Read the model definition and answer for the solid it produces. Units are mm, in the model's axes. A direction names the side the tool comes from. Give positions to 0.01 mm unless a question says otherwise; leave off trailing zeros. Loops run counter-clockwise (first coordinate to the right, second up) from the corner with the lowest first, then second, coordinate; pieces in that order, holes last. Notation, with made-up numbers: (-36.5, 75) - (21.5, 75) arc R25 ccw to (21.5, 94) - close; hole circle Ø9 at (76.5, -20.5). An arc over 180 degrees is marked (long way). Write item = value, one per line.
```python
from build123d import *

# Parameters (mm, degrees)
SKETCH1_W                      = 52.7
SKETCH1_H                      = 40.2
SKETCH1_W_2                    = 40
SKETCH1_H_2                    = 27.5
BOSS_EXTRUDE1_DEPTH            = 46
SKETCH2_R                      = 1.7
SKETCH2_R_2                    = 3.25
CUT_EXTRUDE1_DEPTH             = 6.35
BOSS_EXTRUDE2_DEPTH            = 242.29
SKETCH4_W                      = 288.29
SKETCH4_H                      = 6.35
BOSS_EXTRUDE3_DEPTH            = 7
SKETCH6_W                      = 288.29
SKETCH6_H                      = 6.35
BOSS_EXTRUDE4_DEPTH            = 7
SKETCH7_W                      = 6.35
SKETCH7_H                      = 25
BOSS_EXTRUDE5_DEPTH            = 7
CUT_EXTRUDE2_REACH             = 297.989
SKETCH9_R                      = 2.5
CUT_EXTRUDE2_DIRECTION_2_REACH = 297.989
CUT_EXTRUDE3_REACH             = 253.822
SKETCH10_R                     = 1.2
SKETCH11_W                     = 21.35
SKETCH11_H                     = 6.8
SKETCH11_W_2                   = 214.59
CUT_EXTRUDE4_DEPTH             = 52.7
SKETCH12_W                     = 6.35
SKETCH12_H                     = 6.35
CUT_EXTRUDE5_DEPTH             = 6.8


with BuildPart() as part:
    # Sketch1 → Boss-Extrude1 (new body)
    with BuildSketch(Plane.XY):
        with Locations((20, 13.75)):
            Rectangle(SKETCH1_W, SKETCH1_H)
        with Locations((20, 13.75)):
            Rectangle(SKETCH1_W_2, SKETCH1_H_2, mode=Mode.SUBTRACT)
    extrude(amount=BOSS_EXTRUDE1_DEPTH)

    # Sketch2 → Cut-Extrude1 (cut)
    with BuildSketch(Plane.XZ.offset(6.35)):
        with Locations(Location((29, 39.5, 0), (0, 0, 270))):
            Circle(SKETCH2_R)
        with Locations(Location((11, 39.5, 0), (0, 0, 270))):
            Circle(SKETCH2_R)
        with Locations(Location((11, 6.5, 0), (0, 0, 270))):
            Circle(SKETCH2_R)
        with Locations(Location((29, 6.5, 0), (0, 0, 270))):
            Circle(SKETCH2_R)
        with Locations(Location((20, 30.5, 0), (0, 0, 270))):
            Circle(SKETCH2_R_2)
    extrude(amount=-CUT_EXTRUDE1_DEPTH, mode=Mode.SUBTRACT)

    # Sketch3 → Boss-Extrude2 (add)
    with BuildSketch(Plane(origin=(0, 0, 0), x_dir=(-1, 0, 0), z_dir=(0, 0, -1))):
        Polygon((6.35, 33.85), (6.35, -13.15), (0, -13.15), (0, 27.5), (-40, 27.5), (-40, -13.15), (-46.35, -13.15), (-46.35, 33.85), align=None)
    extrude(amount=BOSS_EXTRUDE2_DEPTH)

    # Sketch4 → Boss-Extrude3 (add)
    with BuildSketch(Plane.ZY.offset(6.35)):
        with Locations((-98.145, 30.675)):
            Rectangle(SKETCH4_W, SKETCH4_H)
    extrude(amount=BOSS_EXTRUDE3_DEPTH)

    # Sketch6 → Boss-Extrude4 (add)
    with BuildSketch(Plane(origin=(46.35, 0, 0), x_dir=(0, 0, -1), z_dir=(1, 0, 0))):
        with Locations((98.145, 30.675)):
            Rectangle(SKETCH6_W, SKETCH6_H)
    extrude(amount=BOSS_EXTRUDE4_DEPTH)

    # Sketch7 → Boss-Extrude5 (add)
    with BuildSketch(Plane(origin=(46.35, 0, 0), x_dir=(0, 0, -1), z_dir=(1, 0, 0))):
        with Locations((217.765, -0.65)):
            Rectangle(SKETCH7_W, SKETCH7_H)
    extrude(amount=BOSS_EXTRUDE5_DEPTH)

    # Cut-Extrude2: up to this face of the body (flat: up to its plane)
    cut_extrude2_end = Plane(part.part.faces().sort_by_distance((46.35, 7.756141986, -99.825781006))[0])
    # Sketch9 → Cut-Extrude2 (cut, up to the picked face)
    with BuildSketch(Plane(origin=(40, 27.5, -242.29), x_dir=(0, 0, 1), z_dir=(-1, 0, 0)), mode=Mode.PRIVATE) as cut_extrude2_sk1:
        with Locations((210.29, -16.925)):
            Circle(SKETCH9_R)
    cut_extrude2_tool1 = split(extrude(cut_extrude2_sk1.sketch, amount=-CUT_EXTRUDE2_REACH, mode=Mode.PRIVATE), bisect_by=cut_extrude2_end, keep=Keep.BOTH, mode=Mode.PRIVATE)
    add(cut_extrude2_tool1.solids().sort_by(Axis((40, 10.575, -32), (1, 0, 0)))[0], mode=Mode.SUBTRACT)

    # Cut-Extrude2 direction 2: up to this face of the body (flat: up to its plane)
    cut_extrude2_direction_2_end = Plane(part.part.faces().sort_by_distance((-6.35, 7.639146283, -101.467245288))[0])
    # Sketch9 → Cut-Extrude2 direction 2 (cut, up to the picked face)
    with BuildSketch(Plane(origin=(40, 27.5, -242.29), x_dir=(0, 0, 1), z_dir=(-1, 0, 0)), mode=Mode.PRIVATE) as cut_extrude2_direction_2_sk1:
        with Locations((210.29, -16.925)):
            Circle(SKETCH9_R)
    cut_extrude2_direction_2_tool1 = split(extrude(cut_extrude2_direction_2_sk1.sketch, amount=CUT_EXTRUDE2_DIRECTION_2_REACH, mode=Mode.PRIVATE), bisect_by=cut_extrude2_direction_2_end, keep=Keep.BOTH, mode=Mode.PRIVATE)
    add(cut_extrude2_direction_2_tool1.solids().sort_by(Axis((40, 10.575, -32), (-1, 0, 0)))[0], mode=Mode.SUBTRACT)

    # Cut-Extrude3: up to this face of the body (flat: up to its plane)
    cut_extrude3_end = Plane(part.part.faces().sort_by_distance((-6.35, 7.634083702, -101.587034491))[0])
    # Sketch10 → Cut-Extrude3 (cut, up to the picked face)
    with BuildSketch(Plane(origin=(46.35, 0, 0), x_dir=(0, 0, -1), z_dir=(1, 0, 0)), mode=Mode.PRIVATE) as cut_extrude3_sk1:
        with Locations((99, 24)):
            Circle(SKETCH10_R)
    cut_extrude3_tool1 = split(extrude(cut_extrude3_sk1.sketch, amount=-CUT_EXTRUDE3_REACH, mode=Mode.PRIVATE), bisect_by=cut_extrude3_end, keep=Keep.BOTH, mode=Mode.PRIVATE)
    # Sketch10 → Cut-Extrude3 (cut, up to the picked face)
    with BuildSketch(Plane(origin=(46.35, 0, 0), x_dir=(0, 0, -1), z_dir=(1, 0, 0)), mode=Mode.PRIVATE) as cut_extrude3_sk2:
        with Locations((99, 12)):
            Circle(SKETCH10_R)
    cut_extrude3_tool2 = split(extrude(cut_extrude3_sk2.sketch, amount=-CUT_EXTRUDE3_REACH, mode=Mode.PRIVATE), bisect_by=cut_extrude3_end, keep=Keep.BOTH, mode=Mode.PRIVATE)
    # Sketch10 → Cut-Extrude3 (cut, up to the picked face)
    with BuildSketch(Plane(origin=(46.35, 0, 0), x_dir=(0, 0, -1), z_dir=(1, 0, 0)), mode=Mode.PRIVATE) as cut_extrude3_sk3:
        with Locations((107, 12)):
            Circle(SKETCH10_R)
    cut_extrude3_tool3 = split(extrude(cut_extrude3_sk3.sketch, amount=-CUT_EXTRUDE3_REACH, mode=Mode.PRIVATE), bisect_by=cut_extrude3_end, keep=Keep.BOTH, mode=Mode.PRIVATE)
    # Sketch10 → Cut-Extrude3 (cut, up to the picked face)
    with BuildSketch(Plane(origin=(46.35, 0, 0), x_dir=(0, 0, -1), z_dir=(1, 0, 0)), mode=Mode.PRIVATE) as cut_extrude3_sk4:
        with Locations((107, 24)):
            Circle(SKETCH10_R)
    cut_extrude3_tool4 = split(extrude(cut_extrude3_sk4.sketch, amount=-CUT_EXTRUDE3_REACH, mode=Mode.PRIVATE), bisect_by=cut_extrude3_end, keep=Keep.BOTH, mode=Mode.PRIVATE)
    add(cut_extrude3_tool1.solids().sort_by(Axis((46.35, 24, -99), (-1, 0, 0)))[0], mode=Mode.SUBTRACT)
    add(cut_extrude3_tool2.solids().sort_by(Axis((46.35, 12, -99), (-1, 0, 0)))[0], mode=Mode.SUBTRACT)
    add(cut_extrude3_tool3.solids().sort_by(Axis((46.35, 12, -107), (-1, 0, 0)))[0], mode=Mode.SUBTRACT)
    add(cut_extrude3_tool4.solids().sort_by(Axis((46.35, 24, -107), (-1, 0, 0)))[0], mode=Mode.SUBTRACT)

    # Sketch11 → Cut-Extrude4 (cut)
    with BuildSketch(Plane(origin=(46.35, 0, 0), x_dir=(0, 0, -1), z_dir=(1, 0, 0))):
        with Locations((231.615, -9.75)):
            Rectangle(SKETCH11_W, SKETCH11_H)
        with Locations((107.295, -9.75)):
            Rectangle(SKETCH11_W_2, SKETCH11_H)
    extrude(amount=-CUT_EXTRUDE4_DEPTH, mode=Mode.SUBTRACT)

    # Sketch12 → Cut-Extrude5 (cut)
    with BuildSketch(Plane.XZ.offset(13.15)):
        with Locations((-3.175, -217.765)):
            Rectangle(SKETCH12_W, SKETCH12_H)
    extrude(amount=-CUT_EXTRUDE5_DEPTH, mode=Mode.SUBTRACT)


solid = part.part
```
1) A tool of negligible diameter and unlimited length cuts with its end or side. For faces 5 (the face through (20.98, -3.22, 27.4)), 6 (the face through (-10, 27.5, -100)), 7 (the face through (20, 33.85, -96)), 8 (the face through (20, -3, 0)), 9 (the face through (20, 0, 23)), from which of +Z, -Z, +X, -X, +Y, -Y can it reach the whole face along a straight path? Write none if from no direction.
Output:
face_5 = -Y
face_6 = +Z, -Z, -X, -Y
face_7 = +Z, -Z, +X, -X, +Y
face_8 = -Z, -Y
face_9 = +Z, -Z
2) A cutting plane is placed at C-C on z = -32. Determine the outline of the cut face in (x, y) (3 decimals), then the cut area to 3 significant figures.
Output:
outline = (-13.35, 27.5) - (-6.35, 27.5) - (-6.35, 13.075) - (0, 13.075) - (0, 27.5) - (40, 27.5) - (40, 13.075) - (46.35, 13.075) - (46.35, 27.5) - (53.35, 27.5) - (53.35, 33.85) - (-13.35, 33.85) - close; (-6.35, -6.35) - (0, -6.35) - (0, 8.075) - (-6.35, 8.075) - close; (40, -6.35) - (46.35, -6.35) - (46.35, 8.075) - (40, 8.075) - close
area = 790 mm²
3) A cutting plane is placed at B-B on x = 20. Determine the outline of the cut face in (y, z), then the cut area to 3 significant figures.
Output:
outline = (-6.35, 0) - (0, 0) - (0, 27.25) - (-6.35, 27.25) - close; (-6.35, 33.75) - (0, 33.75) - (0, 46) - (-6.35, 46) - close; (27.5, -242.29) - (33.85, -242.29) - (33.85, 46) - (27.5, 46) - close
area = 2,080 mm²
4) Each of these flat-tipped pins is pushed along its axis until it touches: P1, Ø5, axis at y = -2, z = -176.5, coming from the +X side; P2, Ø3, axis at y = 24, z = -107, coming from the -X side; P3, Ø5.5, axis at x = -8.5, z = -60.5, coming from the -Y side. Where does it stop, or does it pass through?
Output:
P1 = 46.35
P2 = -6.35
P3 = -6.35
5) Find the intervals of material crossed by probe 1 along Y at (x, z) = (45, -107); probe 2 along X at (y, z) = (7, -138.5); probe 3 along Y at (x, z) = (44.75, -32) (3 decimals), in increasing order.
Output:
probe_1 = -6.35 to 10.8, 13.2 to 22.8, 25.2 to 33.85
probe_2 = -6.35 to 0, 40 to 46.35
probe_3 = -6.35 to 8.075, 13.075 to 33.85
6) A cutting plane is placed at A-A on y = 19. Determine the outline of the cut face in (x, z).
Output:
outline = (-6.35, -242.29) - (0, -242.29) - (0, 46) - (-6.35, 46) - close; (40, -242.29) - (46.35, -242.29) - (46.35, 46) - (40, 46) - close
7) The mould has two halves that part along Y. Classify faces 1 (the face through (50, 11.85, -218)), 2 (the face through (-13.35, 31, -100)), 3 (the face through (43.131, 10.685, -34.498)), 4 (the face through (43, -6.35, -231)): pulls with the +Y half, pulls with the -Y half, needs draft (parallel to the pull), parting line crosses it, or undercut.
Output:
face_1 = undercut
face_2 = needs draft
face_3 = undercut
face_4 = pulls with the -Y half
8) A cutting plane is placed at D-D on x = 34. Determine the outline of the cut face in (y, z), then the cut area to 3 significant figures.
Output:
outline = (-6.35, 0) - (0, 0) - (0, 46) - (-6.35, 46) - close; (27.5, -242.29) - (33.85, -242.29) - (33.85, 46) - (27.5, 46) - close
area = 2,120 mm²
